Check sheet for the modelled part. Datum: model origin and axes. Units: mm. Coordinates: 2 decimals unless noted, no trailing zeros. Loops run counter-clockwise (first coordinate to the right, second up) from the corner with the lowest first, then second, coordinate; pieces in that order, holes last. Notation, with made-up numbers: (19, 36.25) - (73, 36.25) arc R22 ccw to (73, 68.25) - close; hole circle Ø7 at (88.5, -36). An arc over 180 degrees is marked (long way). Use a Markdown table: item, result. Add a question column.
1) Sectioned sample at C-C, the plane y = -11.5. Enter the section's corners in (x, z) (3 decimals).
2) Sectioned sample at A-A, the plane x = 6. Enter the section's corners in (y, z) (3 decimals), then the cut area to 3 significant figures.
3) Go/stop test with flat-tipped pins: P1, Ø4, axis at x = 5.5, y = 12, coming from the -Z side; P2, Ø4, axis at x = 1.5, y = 15, coming from the -Z side. Record where each tip stops, or that it passes through.
4) Sectioned sample at B-B, the plane z = 24. Enter the section's corners in (x, y) (3 decimals), then the cut area to 3 significant figures.
5) Thickness scan on line 1 (Y direction, x = 0.5, z = 39); line 2 (Z direction, x = 7.25, y = 12) (3 decimals); line 3 (Y direction, x = 5, z = 48). Record the ranges inside material, lowest first.
from build123d import *

# Parameters (mm, degrees)
F1_DEPTH = 9.525
F2_R     = 12.7


# Not quite as in the source:
# - a feature names something its author has since deleted; it is built from what else it names


with BuildPart() as f1:
    # F0 (on Right) → F1 (new body)
    with BuildSketch(Plane.YZ):
        Polygon((-19.05, 22.225), (-19.05, -79.375), (19.05, -79.375), (19.05, 79.375), (0, 79.375), align=None)
    extrude(amount=F1_DEPTH)

    # F2
    f2_edges = [f1.edges().sort_by_distance(p)[0] for p in [
        (4.7625, -19.05, -79.375),
        (4.7625, 19.05, -79.375),
    ]]
    fillet(f2_edges, radius=F2_R)


solid = f1.part
Solved:
| question | item | result |
|---|---|---|
| 1 | outline | (0, -78.284) - (9.525, -78.284) - (9.525, 44.875) - (0, 44.875) - close |
| 2 | outline | (-19.05, -66.675) arc R12.7 ccw to (-6.35, -79.375) - (6.35, -79.375) arc R12.7 ccw to (19.05, -66.675) - (19.05, 79.375) - (0, 79.375) - (-19.05, 22.225) - close |
| 2 | area | 5,430 mm2 |
| 3 | P1 | stops at z = -78.84 |
| 3 | P2 | stops at z = -77.49 |
| 4 | outline | (0, -18.458) - (9.525, -18.458) - (9.525, 19.05) - (0, 19.05) - close |
| 4 | area | 357 mm2 |
| 5 | line 1 | y = -13.46 to 19.05 |
| 5 | line 2 | z = -78.049 to 79.375 |
| 5 | line 3 | y = -10.46 to 19.05 |
